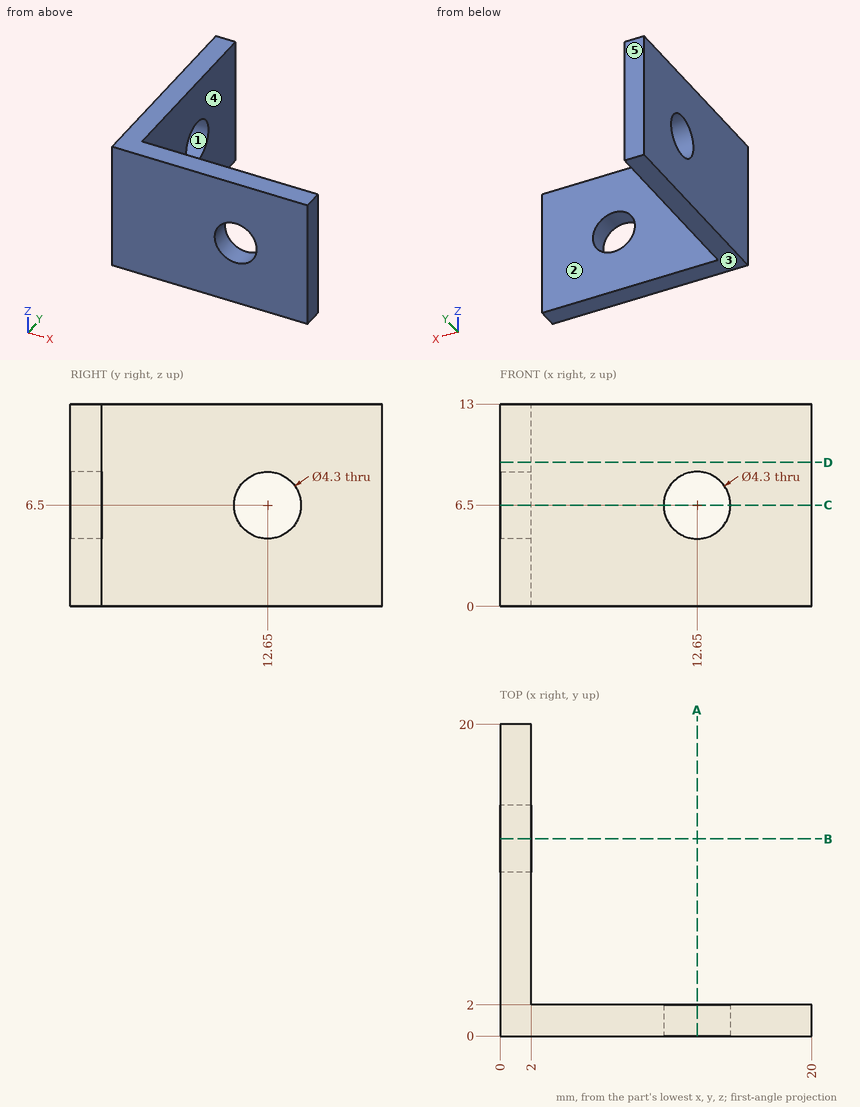
Print and shaded views of the part. All mm, measured from the part's lowest x, y and z. A direction names the side the tool comes from. Coordinates: 2 decimals unless noted, no trailing zeros. Write each loop counter-clockwise with the first axis right and the second up, starting at its lowest first coordinate (ties: lowest second). Pieces come first, ordered by that corner, then holes.
(1) Cut at C-C, the plane z = 6.5. List the corners of the cut face in (x, y), and give its area (3 significant figures).
(2) Two-plate mould, pull along Z, no slides. Class the marked faces 1, 2 and 3: +Z half, -Z half, draft (parallel to the pull), parting line (faces both ways), or undercut.
(3) Drill centre lines: probe 1 along Z at (x, y) = (12.65, 0.65); probe 2 along Y at (x, z) = (0.85, 6.5); probe 3 along Y at (x, z) = (18.75, 11.5). Where is each one in solid material? Low to high.
(4) Cut at D-D, the plane z = 9.25. List the corners of the cut face in (x, y).
(5) 3-axis set-ups, long thin cutter, end or side, ignore diameter. For the marked faces 4 and 5: which of +Z, -Z, +X, -X, +Y, -Y reach the whole face in a straight line?
(6) Cut at A-A, the plane x = 12.65. List the corners of the cut face in (y, z).
(7) Flat gauge pins, fed straight in: pin 1 (3 mm diameter, centred on x = 6.5, z = 4.5, fed in from +Y); pin 2 (6 mm diameter, centred on y = 15, z = 9.5, fed in from -X); pin 3 (4 mm diameter, centred on y = 13.5, z = 6, fed in from +X); pin 4 (4 mm diameter, centred on y = 12.65, z = 6.5, fed in from +X). Where does each tip first touch, or does it go through?
Geometry says:
1. outline: (0, 0) - (10.5, 0) - (10.5, 2) - (2, 2) - (2, 10.5) - (0, 10.5) - close; (0, 14.8) - (2, 14.8) - (2, 20) - (0, 20) - close; (14.8, 0) - (20, 0) - (20, 2) - (14.8, 2) - close
1. area: 58.8 mm2
2. face 1: undercut
2. face 2: draft
2. face 3: -Z half
3. probe 1: z = 0 to 4.35, 8.65 to 13
3. probe 2: y = 0 to 10.5, 14.8 to 20
3. probe 3: y = 0 to 2
4. outline: (0, 0) - (20, 0) - (20, 2) - (2, 2) - (2, 20) - (0, 20) - close
5. face 4: +Z, -Z, +X, +Y
5. face 5: +Z, -Z, +X, -X, +Y
6. outline: (0, 0) - (2, 0) - (2, 4.35) - (0, 4.35) - close; (0, 8.65) - (2, 8.65) - (2, 13) - (0, 13) - close
7. pin 1: stops at y = 2
7. pin 2: stops at x = 0
7. pin 3: stops at x = 2
7. pin 4: passes through
